Geometry: final body of the model. Coordinates: model frame, mm. Face numbers are marked on the shaded views. A direction names the side the tool comes from. Round coordinates to 2 decimals unless told otherwise and drop trailing zeros. Write each loop counter-clockwise with the first axis right and the second up, starting at its lowest first coordinate (ties: lowest second). Pieces come first, ordered by that corner, then holes. Notation, with made-up numbers: M 33,53 L 87,53 A22 cw 87,83 Z; hole C 36.5,45 d4. An arc over 180 degrees is marked long. Use one line per item in the form item = value. Start each with the question number.
Item 1: Section query C-C (z = 7). Return loops of the section in (x, y), and give its area (3 significant figures).
Item 2: Reachability of the marked faces 4 and 5 from +Z, -Z, +X, -X, +Y, -Y: full face, straight path, thin tool, end or side. Return the list, or none.
Item 3: Ray query, probe 1 along X at (y, z) = (241.3, 10.25); probe 2 along Y at (x, z) = (230.5, 28.5); probe 3 along X at (y, z) = (242, 4). Return the intervals inside material, ascending.
Item 4: Section query A-A (y = 241.3). Return loops of the section in (x, z), and give its area (3 significant figures).
Item 5: Section query D-D (y = 250.5). Return loops of the section in (x, z), and give its area (3 significant figures).
Item 6: Pin query (flat end, axial travel): pin 1 Ø1.5 at (x, y) = (231.5, 244) entering from +Z; pin 2 Ø3 at (x, y) = (233, 233.5) entering from +Z. Return the tip coordinate at first contact, or that it passes through.
Item 7: Pull-direction query (X, two-part tool) for the marked faces 1, 2 and 3; classes: pulls with the +X half, pulls with the -X half, needs draft (parallel to the pull), parting line crosses it, or undercut.
Item 8: Section query B-B (x = 225). Return loops of the section in (y, z), and give its area (3 significant figures).
from build123d import *

# Parameters (mm, degrees)
SKETCH1_W           = 57.15
SKETCH1_H           = 25.4
SKETCH1_R           = 2.38125
BOSS_EXTRUDE1_DEPTH = 34.036
SKETCH2_R           = 3.281447176
CUT_EXTRUDE1_DEPTH  = 259.444021221
CUT_EXTRUDE2_DEPTH  = 263.565366711


with BuildPart() as part:
    # Sketch1 → Boss-Extrude1 (new body)
    with BuildSketch(Plane.XY):
        with Locations((226.355780427, 241.3)):
            Rectangle(SKETCH1_W, SKETCH1_H)
        with Locations((245.405780427, 241.3)):
            Circle(SKETCH1_R, mode=Mode.SUBTRACT)
        with Locations((207.305780427, 241.3)):
            Circle(SKETCH1_R, mode=Mode.SUBTRACT)
    extrude(amount=BOSS_EXTRUDE1_DEPTH)

    # Sketch2 → Cut-Extrude1 (cut, through all)
    with BuildSketch(Plane(origin=(0, 254, 0), x_dir=(1, 0, 0), z_dir=(0, 1, 0))):
        with BuildLine():
            Line((254.930780427, -34.036), (254.930780427, -19.05))
            Line((254.930780427, -19.05), (230.6329732, -32.902407479))
            ThreePointArc((230.6329732, -32.902407479), (228.568211783, -33.747792732), (226.355780427, -34.036))
            Line((226.355780427, -34.036), (254.930780427, -34.036))
        make_face()
        with BuildLine():
            Line((197.780780427, -34.036), (226.355780427, -34.036))
            ThreePointArc((226.355780427, -34.036), (224.143349071, -33.747792732), (222.078587654, -32.902407479))
            Line((222.078587654, -32.902407479), (197.780780427, -19.05))
            Line((197.780780427, -19.05), (197.780780427, -34.036))
        make_face()
        Polygon((226.681841891, -42.314106695), (197.780780427, -34.036), (254.930780427, -34.036), align=None)
        with Locations(Location((226.355780427, -25.4, 0), (0, 0, 270))):
            Circle(SKETCH2_R)
    extrude(amount=-CUT_EXTRUDE1_DEPTH, mode=Mode.SUBTRACT)

    # Sketch3 → Cut-Extrude2 (cut, through all)
    with BuildSketch(Plane.ZY.offset(-197.780780427)):
        with BuildLine():
            Line((19.05, 247.65), (49.022, 247.65))
            ThreePointArc((49.022, 247.65), (55.372, 241.3), (49.022, 234.95))
            Line((49.022, 234.95), (19.05, 234.95))
            ThreePointArc((19.05, 234.95), (12.7, 241.3), (19.05, 247.65))
        make_face()
    extrude(amount=-CUT_EXTRUDE2_DEPTH, mode=Mode.SUBTRACT)


solid = part.part
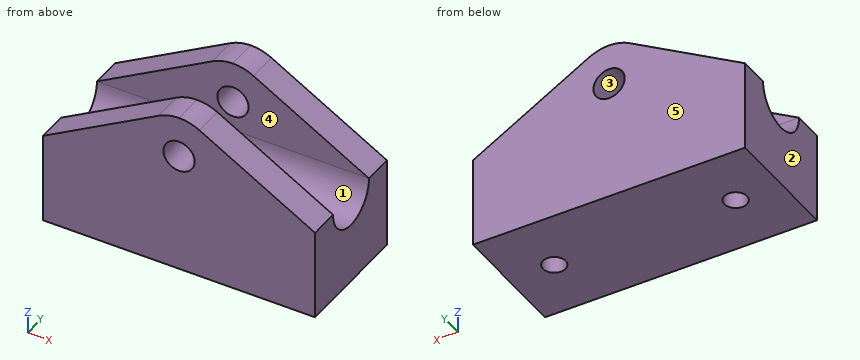
Working result:
q1.outline = M 197.78,228.6 L 254.93,228.6 L 254.93,254 L 197.78,254 Z; hole C 207.31,241.3 d4.76; hole C 245.41,241.3 d4.76
q1.area = 1,420 mm²
q2.face_4 = +Z, +X, -X
q2.face_5 = +Z, -Z, +X, -X, +Y
q3.probe_1 = 197.78 to 204.92, 209.69 to 243.02, 247.79 to 254.93
q3.probe_2 = 228.6 to 234.95, 247.65 to 254
q3.probe_3 = 197.78 to 205.03, 209.58 to 243.13, 247.68 to 254.93
q4.outline = M 197.78,0 L 204.92,0 L 204.92,12.7 L 197.78,12.7 Z; M 209.69,0 L 243.02,0 L 243.02,12.7 L 209.69,12.7 Z; M 247.79,0 L 254.93,0 L 254.93,12.7 L 247.79,12.7 Z
q4.area = 605 mm²
q5.outline = M 197.78,0 L 254.93,0 L 254.93,19.05 L 230.63,32.9 A8.64 ccw 222.08,32.9 L 197.78,19.05 Z; hole C 226.36,25.4 d6.56
q5.area = 1,520 mm²
q6.pin_1 = 13.72
q6.pin_2 = 32.41
q7.face_1 = needs draft
q7.face_2 = pulls with the -X half
q7.face_3 = undercut
q8.outline = M 228.6,0 L 254,0 L 254,22.41 L 247.65,22.41 L 247.65,19.05 A6.35 cw 234.95,19.05 L 234.95,22.41 L 228.6,22.41 Z; M 228.6,28.39 L 234.95,28.39 L 234.95,33.93 L 228.6,33.93 Z; M 247.65,28.39 L 254,28.39 L 254,33.93 L 247.65,33.93 Z
q8.area = 534 mm²
